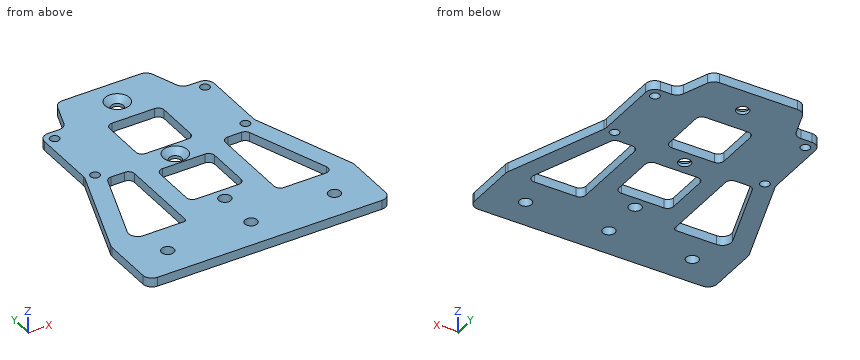
from build123d import *

# Parameters (mm, degrees)
EXTRUDE_1_DEPTH           = 1.5
SKETCH_2_W                = 18
SKETCH_2_H                = 18
CUT_EXTRUDE_1_DEPTH       = 3
FILLET_1_R                = 1
FILLET_2_R                = 2
FILLET_3_R                = 3
SKETCH_3_R                = 2.025
CUT_EXTRUDE_2_DEPTH       = 1
CUT_EXTRUDE_2_DEPTH_BACK  = 4
SKETCH_4_R                = 2.025
CUT_EXTRUDE_3_DEPTH       = 1
CUT_EXTRUDE_3_DEPTH_BACK  = 4
SKETCH_5_R                = 2.025
CUT_EXTRUDE_4_DEPTH       = 1
CUT_EXTRUDE_4_DEPTH_BACK  = 4
FILLET_4_R                = 3
EXTRUDE_2_DEPTH           = 3
FILLET_5_R                = 3
SKETCH_7_R                = 1.525
CUT_EXTRUDE_5_DEPTH       = 3
HOLE_WIZARD_1_D           = 4.05
HOLE_WIZARD_1_DEPTH       = 100
HOLE_WIZARD_1_CSINK_D     = 8
HOLE_WIZARD_1_CSINK_ANGLE = 90
FILLET_6_R                = 2


with BuildPart() as part:
    # 草图1 → 凸台-拉伸1 (new body, symmetric)
    with BuildSketch(Plane.XY):
        Polygon((40, 0), (-40, 0), (-40, 20), (-15, 90), (15, 90), (40, 20), align=None)
    extrude(amount=EXTRUDE_1_DEPTH, both=True)

    # 草图2 → 切除-拉伸1 (cut)
    with BuildSketch(Plane.XY.offset(1.5)):
        Polygon((-15, 72.160717503), (-33.62882768, 20), (-15, 20), align=None)
        with Locations((0, 64)):
            Rectangle(SKETCH_2_W, SKETCH_2_H)
        with Locations((0, 37)):
            Rectangle(SKETCH_2_W, SKETCH_2_H)
        Polygon((15, 20), (15, 72.160717503), (33.62882768, 20), align=None)
    extrude(amount=-CUT_EXTRUDE_1_DEPTH, mode=Mode.SUBTRACT)

    # 圆角1
    fillet_1_edges = [part.edges().sort_by_distance(p)[0] for p in [
        (-15, 20, 0),
        (-15, 72.160717503, 0),
    ]]
    fillet(fillet_1_edges, radius=FILLET_1_R)

    # 圆角2
    fillet_2_edges = [part.edges().sort_by_distance(p)[0] for p in [
        (-9, 46, 0),
        (-9, 28, 0),
        (9, 28, 0),
        (9, 46, 0),
        (-9, 73, 0),
        (-9, 55, 0),
        (9, 55, 0),
        (9, 73, 0),
    ]]
    fillet(fillet_2_edges, radius=FILLET_2_R)

    # 圆角3
    fillet_3_edges = [part.edges().sort_by_distance(p)[0] for p in [
        (40, 0, 0),
        (-40, 0, 0),
        (-40, 20, 0),
        (-15, 90, 0),
        (15, 90, 0),
        (40, 20, 0),
    ]]
    fillet(fillet_3_edges, radius=FILLET_3_R)

    # 草图3 → 切除-拉伸2 (cut, two sides)
    with BuildSketch(Plane.XY.offset(1.5)) as cut_extrude_2_sk:
        with Locations((-27.5, 10)):
            Circle(SKETCH_3_R)
        with Locations((27.5, 10)):
            Circle(SKETCH_3_R)
    extrude(amount=CUT_EXTRUDE_2_DEPTH, mode=Mode.SUBTRACT)
    extrude(cut_extrude_2_sk.sketch, amount=-CUT_EXTRUDE_2_DEPTH_BACK, mode=Mode.SUBTRACT)

    # 草图4 → 切除-拉伸3 (cut, two sides)
    with BuildSketch(Plane.XY.offset(1.5)) as cut_extrude_3_sk:
        with Locations((0, 10)):
            Circle(SKETCH_4_R)
    extrude(amount=CUT_EXTRUDE_3_DEPTH, mode=Mode.SUBTRACT)
    extrude(cut_extrude_3_sk.sketch, amount=-CUT_EXTRUDE_3_DEPTH_BACK, mode=Mode.SUBTRACT)

    # 草图5 → 切除-拉伸4 (cut, two sides)
    with BuildSketch(Plane.XY.offset(1.5)) as cut_extrude_4_sk:
        with Locations((0, 24)):
            Circle(SKETCH_5_R)
        with Locations((0, 50.5)):
            Circle(SKETCH_5_R)
        with Locations((0, 81.5)):
            Circle(SKETCH_5_R)
    extrude(amount=CUT_EXTRUDE_4_DEPTH, mode=Mode.SUBTRACT)
    extrude(cut_extrude_4_sk.sketch, amount=-CUT_EXTRUDE_4_DEPTH_BACK, mode=Mode.SUBTRACT)

    # 圆角4
    fillet_4_edges = [part.edges().sort_by_distance(p)[0] for p in [
        (-33.62882768, 20, 0),
    ]]
    fillet(fillet_4_edges, radius=FILLET_4_R)

    # 草图6 → 凸台-拉伸2 (add)
    with BuildSketch(Plane(origin=(0, 0, -1.5), x_dir=(-1, 0, 0), z_dir=(0, 0, -1))):
        Polygon((-28, 78), (-28, 53.6), (-19.285714286, 78), align=None)
        Polygon((28, 78), (19.285714286, 78), (28, 53.6), align=None)
        Polygon((-15, 72.160717503), (-22.914541965, 50), (-15, 50), align=None)
        with BuildLine():
            Line((15, 66.387503754), (15, 50))
            Line((15, 50), (22.914541965, 50))
            Line((22.914541965, 50), (16.941741912, 66.723840151))
            ThreePointArc((16.941741912, 66.723840151), (15.82932767, 67.372831596), (15, 66.387503754))
        make_face()
    extrude(amount=-EXTRUDE_2_DEPTH)

    # 圆角5
    fillet_5_edges = [part.edges().sort_by_distance(p)[0] for p in [
        (28, 78, 0),
        (19.285714286, 78, 0),
        (28, 53.6, 0),
        (-28, 78, 0),
        (-19.285714286, 78, 0),
        (-28, 53.6, 0),
    ]]
    fillet(fillet_5_edges, radius=FILLET_5_R)

    # 草图7 → 切除-拉伸5 (cut)
    with BuildSketch(Plane(origin=(0, 0, -1.5), x_dir=(-1, 0, 0), z_dir=(0, 0, -1))):
        with Locations((24.8, 74.8)):
            Circle(SKETCH_7_R)
        with Locations((24.8, 53.2)):
            Circle(SKETCH_7_R)
        with Locations((-24.8, 53.2)):
            Circle(SKETCH_7_R)
        with Locations((-24.8, 74.8)):
            Circle(SKETCH_7_R)
    extrude(amount=-CUT_EXTRUDE_5_DEPTH, mode=Mode.SUBTRACT)

    # 孔1
    with Locations(Plane.XY.offset(1.5)):
        with Locations((0, 81.5), (0, 50.5)):
            CounterSinkHole(HOLE_WIZARD_1_D / 2, HOLE_WIZARD_1_CSINK_D / 2, depth=HOLE_WIZARD_1_DEPTH, counter_sink_angle=HOLE_WIZARD_1_CSINK_ANGLE)

    # 圆角6
    fillet_6_edges = [part.edges().sort_by_distance(p)[0] for p in [
        (15, 50, 0),
        (22.914541965, 50, 0),
        (-22.914541965, 50, 0),
        (-15, 50, 0),
        (15, 20, 0),
        (33.62882768, 20, 0),
    ]]
    fillet(fillet_6_edges, radius=FILLET_6_R)


solid = part.part
Design review of the part built by this model. Coordinates are the model's own, in mm. Give positions to 0.01 mm unless a question says otherwise; leave off trailing zeros. Loops run counter-clockwise (first coordinate to the right, second up) from the corner with the lowest first, then second, coordinate; pieces in that order, holes last. Notation, with made-up numbers: (24.5, 85) - (71.5, 85) arc R14 cw to (71.5, 104) - close; hole circle Ø11 at (0.5, 49.25). An arc over 180 degrees is marked (long way). Write item = value, one per line.
1) Clearance check with flat-ended pins moving along their axes: pin 1 Ø1.5 at (y, z) = (37, -0.5) entering from -X; pin 2 Ø1.5 at (y, z) = (38.5, 0) entering from +X; pin 3 Ø0.9 at (y, z) = (65.5, 0.5) entering from -X. State where each tip first meets the part, or that it passes through.
Result sheet:
pin_1 = -34.2
pin_2 = 33.66
pin_3 = -28
2) Take a section at C-C on y = 39. State the section outline as (x, z) points.
Result sheet:
outline = (-33.21, -1.5) - (-26.84, -1.5) - (-26.84, 1.5) - (-33.21, 1.5) - close; (-15, -1.5) - (-9, -1.5) - (-9, 1.5) - (-15, 1.5) - close; (9, -1.5) - (15, -1.5) - (15, 1.5) - (9, 1.5) - close; (26.84, -1.5) - (33.21, -1.5) - (33.21, 1.5) - (26.84, 1.5) - close
3) Take a section at A-A on y = 10. State the section outline as (x, z) points (3 decimals), and give its area (3 significant figures).
Result sheet:
outline = (-40, -1.5) - (-29.525, -1.5) - (-29.525, 1.5) - (-40, 1.5) - close; (-25.475, -1.5) - (-2.025, -1.5) - (-2.025, 1.5) - (-25.475, 1.5) - close; (2.025, -1.5) - (25.475, -1.5) - (25.475, 1.5) - (2.025, 1.5) - close; (29.525, -1.5) - (40, -1.5) - (40, 1.5) - (29.525, 1.5) - close
area = 204 mm2
4) To check wall thickness, follow line 1 (X direction, y = 74.8, z = -0.8) (3 decimals); line 2 (Y direction, x = 8, z = -0.2); line 3 (X direction, y = 38, z = 0.9). State the ranges of each line that lie inside material, in increasing order.
Result sheet:
line_1 = -28 to -26.325, -23.275 to 23.275, 26.325 to 28
line_2 = 0 to 28.27, 45.73 to 55.27, 72.73 to 90
line_3 = -33.57 to -27.2, -15 to -9, 9 to 15, 27.2 to 33.57
5) Take a section at B-B on x = 0. Count the separate pieces of the cut face and the enclosed holes in it, and give its area (3 significant figures).
Result sheet:
separate_pieces = 7
enclosed_holes = 0
area = 106 mm2
